Design review of the part shown in the three views and the two pictorial views. Dimensions are in mm from the part's minimum x, y and z. Coordinates: 2 decimals unless noted, no trailing zeros. Write each loop counter-clockwise with the first axis right and the second up, starting at its lowest first coordinate (ties: lowest second). Pieces come first, ordered by that corner, then holes. Notation, with made-up numbers: (23, 19.5) - (42, 19.5) arc R6 ccw to (42, 25.5) - close; hole circle Ø7 at (65.25, -30.5). An arc over 180 degrees is marked (long way). Write each question's results on one line, items separated by ' | '.
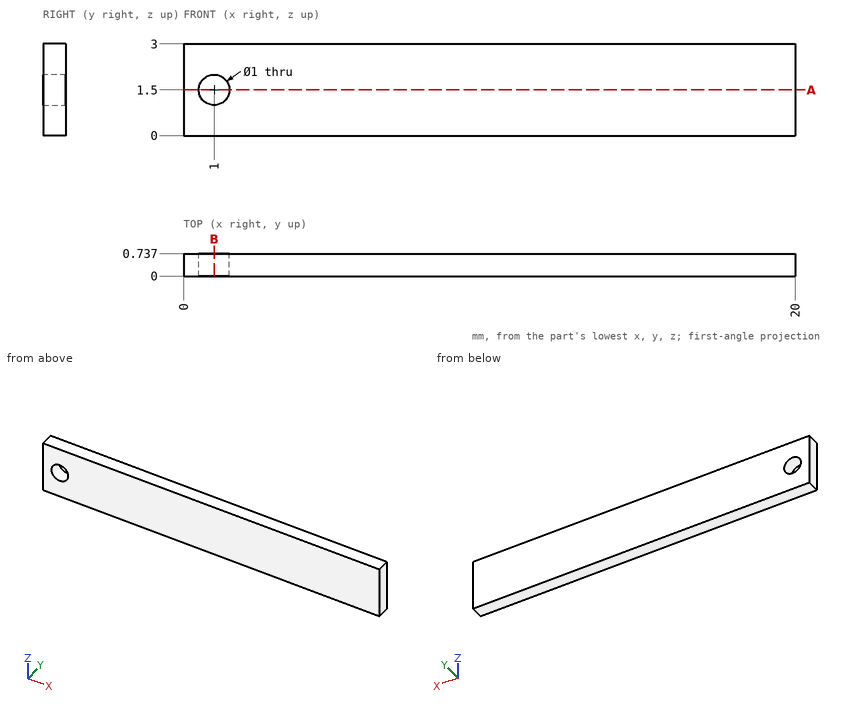
Q1. Take a section at A-A on z = 1.5. State the section outline as (x, y) points, plus the area to 3 significant figures.
Results found:
outline: (0, 0) - (0.5, 0) - (0.5, 0.74) - (0, 0.74) - close; (1.5, 0) - (20, 0) - (20, 0.74) - (1.5, 0.74) - close | area: 14.0 mm2
Q2. Take a section at B-B on x = 1. State the section outline as (y, z) points.
Results found:
outline: (0, 0) - (0.74, 0) - (0.74, 1) - (0, 1) - close; (0, 2) - (0.74, 2) - (0.74, 3) - (0, 3) - close
Q3. Wall thickness on line 1 along X through (y, z) = (0.3, 1.5); line 2 along X through (y, z) = (0.5, 1.2): over which ranges is each line inside the solid? List them lowest first. Write a range as from..to.
Results found:
line 1: 0..0.5, 1.5..20 | line 2: 0..0.6, 1.4..20
